from build123d import *

# Parameters (mm, degrees)
F0_W     = 100
F0_H     = 200
F0_R     = 4.25
F1_DEPTH = 27


with BuildPart() as f1:
    # F0 (on Top) → F1 (new body)
    with BuildSketch(Plane.XY):
        with Locations((-452.313822, 147.181731)):
            Rectangle(F0_W, F0_H)
        with Locations((-489.163222, 63.681799)):
            Circle(F0_R, mode=Mode.SUBTRACT)
        with Locations((-489.179955, 82.181791)):
            Circle(F0_R, mode=Mode.SUBTRACT)
        with Locations((-470.663222, 63.681799)):
            Circle(F0_R, mode=Mode.SUBTRACT)
        with Locations((-470.679955, 82.181791)):
            Circle(F0_R, mode=Mode.SUBTRACT)
        with Locations((-489.196689, 100.681784)):
            Circle(F0_R, mode=Mode.SUBTRACT)
        with Locations((-489.213422, 119.181776)):
            Circle(F0_R, mode=Mode.SUBTRACT)
        with Locations((-489.230155, 137.681768)):
            Circle(F0_R, mode=Mode.SUBTRACT)
        with Locations((-470.696689, 100.681784)):
            Circle(F0_R, mode=Mode.SUBTRACT)
        with Locations((-470.713422, 119.181776)):
            Circle(F0_R, mode=Mode.SUBTRACT)
        with Locations((-470.730155, 137.681768)):
            Circle(F0_R, mode=Mode.SUBTRACT)
        with Locations((-452.163222, 63.681799)):
            Circle(F0_R, mode=Mode.SUBTRACT)
        with Locations((-433.663222, 63.681799)):
            Circle(F0_R, mode=Mode.SUBTRACT)
        with Locations((-452.179955, 82.181791)):
            Circle(F0_R, mode=Mode.SUBTRACT)
        with Locations((-433.679955, 82.181791)):
            Circle(F0_R, mode=Mode.SUBTRACT)
        with Locations((-415.163222, 63.681799)):
            Circle(F0_R, mode=Mode.SUBTRACT)
        with Locations((-415.179955, 82.181791)):
            Circle(F0_R, mode=Mode.SUBTRACT)
        with Locations((-452.196689, 100.681784)):
            Circle(F0_R, mode=Mode.SUBTRACT)
        with Locations((-452.213422, 119.181776)):
            Circle(F0_R, mode=Mode.SUBTRACT)
        with Locations((-433.696689, 100.681784)):
            Circle(F0_R, mode=Mode.SUBTRACT)
        with Locations((-433.713422, 119.181776)):
            Circle(F0_R, mode=Mode.SUBTRACT)
        with Locations((-452.230155, 137.681768)):
            Circle(F0_R, mode=Mode.SUBTRACT)
        with Locations((-433.730155, 137.681768)):
            Circle(F0_R, mode=Mode.SUBTRACT)
        with Locations((-415.196689, 100.681784)):
            Circle(F0_R, mode=Mode.SUBTRACT)
        with Locations((-415.213422, 119.181776)):
            Circle(F0_R, mode=Mode.SUBTRACT)
        with Locations((-415.230155, 137.681768)):
            Circle(F0_R, mode=Mode.SUBTRACT)
        with Locations((-489.246889, 156.181761)):
            Circle(F0_R, mode=Mode.SUBTRACT)
        with Locations((-489.263622, 174.681753)):
            Circle(F0_R, mode=Mode.SUBTRACT)
        with Locations((-489.280356, 193.181746)):
            Circle(F0_R, mode=Mode.SUBTRACT)
        with Locations((-470.746889, 156.181761)):
            Circle(F0_R, mode=Mode.SUBTRACT)
        with Locations((-470.763622, 174.681753)):
            Circle(F0_R, mode=Mode.SUBTRACT)
        with Locations((-470.780356, 193.181746)):
            Circle(F0_R, mode=Mode.SUBTRACT)
        with Locations((-489.297089, 211.681738)):
            Circle(F0_R, mode=Mode.SUBTRACT)
        with Locations((-489.313822, 230.181731)):
            Circle(F0_R, mode=Mode.SUBTRACT)
        with Locations((-470.797089, 211.681738)):
            Circle(F0_R, mode=Mode.SUBTRACT)
        with Locations((-470.813822, 230.181731)):
            Circle(F0_R, mode=Mode.SUBTRACT)
        with Locations((-452.313822, 230.181731)):
            Circle(F0_R, mode=Mode.SUBTRACT)
        with Locations((-452.246889, 156.181761)):
            Circle(F0_R, mode=Mode.SUBTRACT)
        with Locations((-433.746889, 156.181761)):
            Circle(F0_R, mode=Mode.SUBTRACT)
        with Locations((-452.263622, 174.681753)):
            Circle(F0_R, mode=Mode.SUBTRACT)
        with Locations((-452.280356, 193.181746)):
            Circle(F0_R, mode=Mode.SUBTRACT)
        with Locations((-433.763622, 174.681753)):
            Circle(F0_R, mode=Mode.SUBTRACT)
        with Locations((-433.780356, 193.181746)):
            Circle(F0_R, mode=Mode.SUBTRACT)
        with Locations((-415.246889, 156.181761)):
            Circle(F0_R, mode=Mode.SUBTRACT)
        with Locations((-415.263622, 174.681753)):
            Circle(F0_R, mode=Mode.SUBTRACT)
        with Locations((-415.280356, 193.181746)):
            Circle(F0_R, mode=Mode.SUBTRACT)
        with Locations((-452.297089, 211.681738)):
            Circle(F0_R, mode=Mode.SUBTRACT)
        with Locations((-433.797089, 211.681738)):
            Circle(F0_R, mode=Mode.SUBTRACT)
        with Locations((-433.813822, 230.181731)):
            Circle(F0_R, mode=Mode.SUBTRACT)
        with Locations((-415.297089, 211.681738)):
            Circle(F0_R, mode=Mode.SUBTRACT)
        with Locations((-415.313822, 230.181731)):
            Circle(F0_R, mode=Mode.SUBTRACT)
    extrude(amount=F1_DEPTH)


solid = f1.part
Geometry: final body of the model. Coordinates: model frame, mm. Round coordinates to 2 decimals unless told otherwise and drop trailing zeros.
Q1. Mould query, pull axis Y, two halves, no side actions, for faces 1 (the face through (-453, 247.182, 13)), 2 (the face through (-468.479, 178.265, 13.311)), 3 (the face through (-453, 149, 0)). Classes: released by +Y, released by -Y, zero draft, split by the parting line, or undercut.
Result sheet:
face 1: released by +Y
face 2: undercut
face 3: zero draft
Q2. Material intervals for probe 1 along X at (y, z) = (215.5, 20.25); probe 2 along X at (y, z) = (83, 19.5), sorted ascending.
Result sheet:
probe 1: x = -502.31 to -491.16, -487.43 to -472.66, -468.93 to -454.16, -450.43 to -435.66, -431.93 to -417.16, -413.43 to -402.31
probe 2: x = -502.31 to -493.35, -485.01 to -474.85, -466.51 to -456.35, -448.01 to -437.85, -429.51 to -419.35, -411.01 to -402.31
Q3. Section A-A, the plane x = -471. Give the number of separate pieces and of enclosed holes in the cut face, and give its area (3 significant figures).
Result sheet:
separate pieces: 11
enclosed holes: 0
area: 3,110 mm2
